Geometry check sheet. Reference: the model listing, model coordinates, mm. A direction names the side the tool comes from. Round coordinates to 2 decimals unless told otherwise and drop trailing zeros. Loops run counter-clockwise (first coordinate to the right, second up) from the corner with the lowest first, then second, coordinate; pieces in that order, holes last. Notation, with made-up numbers: M 30.5,86.25 L 64.5,86.25 A17 cw 64.5,109.25 Z; hole C 49.25,69.25 d11. An arc over 180 degrees is marked long. Use one line per item in the form item = value. Start each with the question number.
1. Cross-section at A-A (x = 9). Record the boundary of the cut face in (y, z), then the cut area to 3 significant figures.
2. Cross-section at C-C (x = 28). Record the boundary of the cut face in (y, z), then the cut area to 3 significant figures.
3. Cross-section at B-B (y = 3.25). State how many separate pieces and enclosed holes the cut face has, then the cut area to 3 significant figures.
4. Material ranges on line 1 (X direction, y = -0.75, z = 8.5); line 2 (X direction, y = 6, z = 3.5); line 3 (Z direction, x = 26.5, y = -4.75), recorded low to high.
5. Cross-section at D-D (x = -34.5). Record the boundary of the cut face in (y, z), then the cut area to 3 significant figures.
6. Set-up check for faces 1 (the cylindrical face through (39.2, 4.6, 1.1)), 2 (the cylindrical face through (38.42, 0.1, -0.74)), 3 (the flat face through (52, 0, 11)), 4 (the cylindrical face through (-16, -6, -6)), 5 (the cylindrical face through (-1.57, 0.14, 14.15)): record each of +Z, -Z, +X, -X, +Y, -Y from which the full face is reachable in a straight line by a thin tool's end or side.
7. Draft check along Z on faces 6 (the cylindrical face through (0.24, 0.14, -1.87)), 7 (the flat face through (46.915, 4.751, -5.3)), 8 (the flat face through (-45, 10, -11)). Enter one of: pulls with the +Z half, pulls with the -Z half, needs draft (parallel to the pull), parting line crosses it, or undercut.
8. Go/stop test with flat-tipped pins: pin 1 (1.5 mm diameter, centred on x = 27.5, y = 7, fed in from -Z); pin 2 (12 mm diameter, centred on x = 40, z = 5.5, fed in from +Y); pin 3 (1 mm diameter, centred on y = 1.5, z = -14, fed in from -X); pin 4 (10 mm diameter, centred on x = -4.5, z = -9.5, fed in from -Y). Record where each tip stops, or that it passes through.
```python
from build123d import *

# Parameters (mm, degrees)
CROQUIS1_R              = 3.5
SALIENTE_EXTRUIR1_DEPTH = 2
CROQUIS2_R              = 3.5
SALIENTE_EXTRUIR2_DEPTH = 10
SALIENTE_EXTRUIR3_DEPTH = 7
CORTAR_EXTRUIR1_DEPTH   = 83.665164829


with BuildPart() as part:
    # Croquis1 → Saliente-Extruir1 (new, symmetric)
    with BuildSketch(Plane(origin=(0, 0, 0), x_dir=(1, 0, 0), z_dir=(0, 1, 0))):
        with BuildLine():
            Line((-65, 15), (-40.296472568, 15))
            ThreePointArc((-40.296472568, 15), (-25.597104262, 12.999326141), (-11.967141117, 7.142857143))
            ThreePointArc((-11.967141117, 7.142857143), (0.423734469, 1.818794417), (13.786796564, 0))
            Line((13.786796564, 0), (34.644660941, 0))
            ThreePointArc((34.644660941, 0), (38.471495264, 0.761204675), (41.715728753, 2.928932188))
            Line((41.715728753, 2.928932188), (49.393398282, 10.606601718))
            ThreePointArc((49.393398282, 10.606601718), (51.940505875, 12.650871687), (54.86969785, 14.095389312))
            Line((54.86969785, 14.095389312), (55.553738137, 12.21600407))
            ThreePointArc((55.553738137, 12.21600407), (57.74257369, 12.802500789), (60, 13))
            Line((60, 13), (60, 15))
            ThreePointArc((60, 15), (74.095389312, 5.13030215), (69.641814145, -11.490666647))
            Line((69.641814145, -11.490666647), (68.356238926, -9.958577761))
            ThreePointArc((68.356238926, -9.958577761), (66.5, -11.258330249), (64.446261863, -12.21600407))
            Line((64.446261863, -12.21600407), (65.13030215, -14.095389312))
            ThreePointArc((65.13030215, -14.095389312), (62.604722665, -14.772116295), (60, -15))
            Line((60, -15), (21, -15))
            ThreePointArc((21, -15), (-1.892838305, -14.125254625), (-24.652173913, -11.506119696))
            ThreePointArc((-24.652173913, -11.506119696), (-25.259003924, -11.168852013), (-25.5, -10.517765963))
            Line((-25.5, -10.517765963), (-25.5, 10))
            Line((-25.5, 10), (-66, 10))
            Line((-66, 10), (-66, -9))
            ThreePointArc((-66, -9), (-66.292893219, -9.707106781), (-67, -10))
            Line((-67, -10), (-70, -10))
            ThreePointArc((-70, -10), (-73.535533906, -8.535533906), (-75, -5))
            Line((-75, -5), (-75, 5))
            ThreePointArc((-75, 5), (-72.071067812, 12.071067812), (-65, 15))
        make_face()
        with Locations(Location((66.108002035, 2.223130932, 0), (0, 0, 270))):
            Circle(CROQUIS1_R, mode=Mode.SUBTRACT)
        with BuildLine():
            Line((57.461693581, 6.97393957), (62.538306419, -6.97393957))
            ThreePointArc((62.538306419, -6.97393957), (62.17668469, -9.720729309), (59.719228557, -11))
            Line((59.719228557, -11), (43.108950141, -11))
            ThreePointArc((43.108950141, -11), (39.413432011, -8.530733729), (40.280523016, -4.171572875))
            Line((40.280523016, -4.171572875), (52.521295375, 8.069199484))
            ThreePointArc((52.521295375, 8.069199484), (55.29193456, 8.876767161), (57.461693581, 6.97393957))
        make_face(mode=Mode.SUBTRACT)
    extrude(amount=SALIENTE_EXTRUIR1_DEPTH, both=True)

    # Croquis2 → Saliente-Extruir2 (add, symmetric)
    with BuildSketch(Plane(origin=(0, 0, 0), x_dir=(1, 0, 0), z_dir=(0, 1, 0))):
        with BuildLine():
            Line((54.86969785, 14.095389312), (55.553738137, 12.21600407))
            ThreePointArc((55.553738137, 12.21600407), (72.21600407, 4.446261863), (64.446261863, -12.21600407))
            Line((64.446261863, -12.21600407), (65.13030215, -14.095389312))
            ThreePointArc((65.13030215, -14.095389312), (62.604722665, -14.772116295), (60, -15))
            Line((60, -15), (21, -15))
            ThreePointArc((21, -15), (-1.892838305, -14.125254625), (-24.652173913, -11.506119696))
            ThreePointArc((-24.652173913, -11.506119696), (-25.259003924, -11.168852013), (-25.5, -10.517765963))
            Line((-25.5, -10.517765963), (-25.5, 10))
            Line((-25.5, 10), (-66, 10))
            Line((-66, 10), (-66, -9))
            ThreePointArc((-66, -9), (-66.292893219, -9.707106781), (-67, -10))
            Line((-67, -10), (-70, -10))
            ThreePointArc((-70, -10), (-73.535533906, -8.535533906), (-75, -5))
            Line((-75, -5), (-75, 5))
            ThreePointArc((-75, 5), (-72.071067812, 12.071067812), (-65, 15))
            Line((-65, 15), (-40.296472568, 15))
            ThreePointArc((-40.296472568, 15), (-25.597104262, 12.999326141), (-11.967141117, 7.142857143))
            ThreePointArc((-11.967141117, 7.142857143), (0.423734469, 1.818794417), (13.786796564, 0))
            Line((13.786796564, 0), (34.644660941, 0))
            ThreePointArc((34.644660941, 0), (38.471495264, 0.761204675), (41.715728753, 2.928932188))
            Line((41.715728753, 2.928932188), (49.393398282, 10.606601718))
            ThreePointArc((49.393398282, 10.606601718), (51.940505875, 12.650871687), (54.86969785, 14.095389312))
        make_face()
        with Locations(Location((66.108002035, 2.223130932, 0), (0, 0, 270))):
            Circle(CROQUIS2_R, mode=Mode.SUBTRACT)
        with BuildLine():
            Line((13.786796564, -2), (34.644660941, -2))
            ThreePointArc((34.644660941, -2), (39.236862129, -1.08655439), (43.129942315, 1.514718626))
            Line((43.129942315, 1.514718626), (50.807611845, 9.192388155))
            ThreePointArc((50.807611845, 9.192388155), (51.432121169, 9.777088132), (52.093735288, 10.319446608))
            ThreePointArc((52.093735288, 10.319446608), (54.758810503, 10.817874623), (56.737335776, 8.964096282))
            Line((56.737335776, 8.964096282), (63.262664224, -8.964096282))
            ThreePointArc((63.262664224, -8.964096282), (62.938611682, -11.65594441), (60.57666227, -12.987203726))
            ThreePointArc((60.57666227, -12.987203726), (60.288402114, -12.996800538), (60, -13))
            Line((60, -13), (21, -13))
            ThreePointArc((21, -13), (2.813818289, -12.444554152), (-15.304568528, -10.780287213))
            ThreePointArc((-15.304568528, -10.780287213), (-16.872354309, -9.955498637), (-17.5, -8.298908965))
            Line((-17.5, -8.298908965), (-17.5, 3.707419))
            ThreePointArc((-17.5, 3.707419), (-16.248849159, 5.87314654), (-13.747699378, 5.871152614))
            ThreePointArc((-13.747699378, 5.871152614), (-13.371589613, 5.651403898), (-12.997298625, 5.428571429))
            ThreePointArc((-12.997298625, 5.428571429), (-0.110788015, -0.108453806), (13.786796564, -2))
        make_face(mode=Mode.SUBTRACT)
    extrude(amount=SALIENTE_EXTRUIR2_DEPTH, both=True)

    # Croquis3 → Saliente-Extruir3 (add, symmetric)
    with BuildSketch(Plane(origin=(0, 0, 0), x_dir=(1, 0, 0), z_dir=(0, 1, 0))):
        with BuildLine():
            Line((69.641814145, -11.490666647), (68.356238926, -9.958577761))
            ThreePointArc((68.356238926, -9.958577761), (72.21600407, 4.446261863), (60, 13))
            Line((60, 13), (60, 15))
            ThreePointArc((60, 15), (74.095389312, 5.13030215), (69.641814145, -11.490666647))
        make_face()
    extrude(amount=SALIENTE_EXTRUIR3_DEPTH, both=True)

    # Croquis4 → Cortar-Extruir1 (cut, through all, along a direction that is not the sketch's normal)
    with BuildSketch(Plane.XY.offset(15)):
        with BuildLine():
            Line((60, 10), (-10, 10))
            ThreePointArc((-10, 10), (-3.285105416, 9.849625261), (3.416325828, 9.398802543))
            Line((3.416325828, 9.398802543), (33.740168262, 6.675657889))
            ThreePointArc((33.740168262, 6.675657889), (41.229778106, 6.566394932), (48.651667745, 7.577210532))
            Line((48.651667745, 7.577210532), (60, 10))
        make_face()
        with BuildLine():
            Line((60, -10), (-10, -10))
            ThreePointArc((-10, -10), (-3.285105416, -9.849625261), (3.416325828, -9.398802543))
            Line((3.416325828, -9.398802543), (33.740168262, -6.675657889))
            ThreePointArc((33.740168262, -6.675657889), (41.229778106, -6.566394932), (48.651667745, -7.577210532))
            Line((48.651667745, -7.577210532), (60, -10))
        make_face()
    extrude(amount=-CORTAR_EXTRUIR1_DEPTH, dir=(0.1736481776669275, 0, 0.9848077530122086), mode=Mode.SUBTRACT)


solid = part.part
```
Reported:
q1.outline = M -8.89,14.76 L -8.86,12.76 L -2,12.76 L -2,1.78 L -8.69,1.78 L -8.66,-0.23 L 8.66,-0.23 L 8.69,1.78 L 2,1.78 L 2,12.76 L 8.86,12.76 L 8.89,14.76 Z
q1.area = 114 mm²
q2.outline = M -7.19,15 L -7.16,13 L -2,13 L -2,2 L -6.99,2 L -6.95,0 L 6.95,0 L 6.99,2 L 2,2 L 2,13 L 7.16,13 L 7.19,15 Z
q2.area = 101 mm²
q3.separate_pieces = 1
q3.enclosed_holes = 2
q3.area = 1,210 mm²
q4.line_1 = -73.57 to -66, -25.5 to 39.4, 62.68 to 72.36
q4.line_2 = -75 to -66, -25.5 to -17.5, 61.27 to 74.59
q4.line_3 = 0 to 2, 13 to 15
q5.outline = M -10,-14.69 L 10,-14.69 L 10,-10 L -10,-10 Z
q5.area = 93.9 mm²
q6.face_1 = +Y
q6.face_2 = -Z, +Y, -Y
q6.face_3 = +Y, -Y
q6.face_4 = -Y
q6.face_5 = +Z, -X, +Y, -Y
q7.face_6 = pulls with the -Z half
q7.face_7 = undercut
q7.face_8 = needs draft
q8.pin_1 = 0
q8.pin_2 = 6.85
q8.pin_3 = -70.27
q8.pin_4 = through
